```python
from build123d import *

# Parameters (mm, degrees)
ESTRUSIONE_ESTRUSIONE2_DEPTH = 1.6


with BuildPart() as part:
    # bordo2 → Estrusione-Estrusione2 (new body)
    with BuildSketch(Plane.XY):
        with BuildLine():
            Line((201, 97.893856635), (201, -7.091597346))
            ThreePointArc((201, -7.091597346), (198.656854249, -12.748451596), (193, -15.091597346))
            Line((193, -15.091597346), (117.750790543, -15.091597346))
            ThreePointArc((117.750790543, -15.091597346), (116.336576981, -14.505810909), (115.750790543, -13.091597346))
            Line((115.750790543, -13.091597346), (115.750790543, -12.967534141))
            ThreePointArc((115.750790543, -12.967534141), (115.127499694, -11.516785399), (113.64611863, -10.970275071))
            Line((113.64611863, -10.970275071), (0.928841556, -16.877537249))
            ThreePointArc((0.928841556, -16.877537249), (-0.145141858, -16.910699844), (-1.219558299, -16.897682863))
            Line((-1.219558299, -16.897682863), (-151.023233988, -11.861429997))
            ThreePointArc((-151.023233988, -11.861429997), (-156.505538032, -9.426954116), (-158.754433684, -3.865947122))
            Line((-158.754433684, -3.865947122), (-158.754433684, 95.67986032))
            Line((-158.754433684, 95.67986032), (-158.754433684, 110.187089821))
            ThreePointArc((-158.754433684, 110.187089821), (-154.068142183, 121.50079832), (-142.754433684, 126.187089821))
            Line((-142.754433684, 126.187089821), (-39, 126.187089821))
            ThreePointArc((-39, 126.187089821), (-33.343145751, 123.843944071), (-31, 118.187089821))
            Line((-31, 118.187089821), (-31, 105.006491693))
            ThreePointArc((-31, 105.006491693), (-28.802994968, 99.499655087), (-23.41868765, 97.017455415))
            Line((-23.41868765, 97.017455415), (-2.104671912, 95.900435182))
            ThreePointArc((-2.104671912, 95.900435182), (-0.623290849, 96.44694551), (0, 97.897694252))
            Line((0, 97.897694252), (0, 100.897694252))
            ThreePointArc((0, 100.897694252), (0.549251258, 102.274403403), (1.895328088, 102.894953321))
            Line((1.895328088, 102.894953321), (97.91868765, 107.927324355))
            ThreePointArc((97.91868765, 107.927324355), (103.302994968, 110.409524028), (105.5, 115.916360633))
            Line((105.5, 115.916360633), (105.5, 126))
            ThreePointArc((105.5, 126), (107.843145751, 131.656854249), (113.5, 134))
            Line((113.5, 134), (169.851790543, 134))
            ThreePointArc((169.851790543, 134), (172.680217668, 132.828427125), (173.851790543, 130))
            Line((173.851790543, 130), (173.851790543, 130.276535982))
            ThreePointArc((173.851790543, 130.276535982), (175.023363418, 127.448108857), (177.851790543, 126.276535982))
            Line((177.851790543, 126.276535982), (185, 126.276535982))
            ThreePointArc((185, 126.276535982), (196.313708499, 121.590244481), (201, 110.276535982))
            Line((201, 110.276535982), (201, 97.893856635))
        make_face()
    extrude(amount=ESTRUSIONE_ESTRUSIONE2_DEPTH)


solid = part.part
```
The listing builds one solid part. Answer for the finished solid, in the listing's coordinates (mm). A direction names the side the tool comes from. Round coordinates to 2 decimals unless told otherwise and drop trailing zeros. Loops run counter-clockwise (first coordinate to the right, second up) from the corner with the lowest first, then second, coordinate; pieces in that order, holes last.
Q1. Which of the six approach directions +Z, -Z, +X, -X, +Y, -Y give full straight-line access (tool end or side, diameter ignored) to faces 1 (the face through (103.244, 110.348, 0.789)), 2 (the face through (58.077, -13.883, 0.789)), 3 (the face through (-156.445, -9.489, 0.789))?
Q2. Find the intervals of material crossed by line 1 (X direction, y = 110, z = 1.55); line 2 (Y direction, x = 168, z = 0.5); line 3 (Y direction, x = -55.5, z = 0.5), in increasing order.
Q3. Section B-B, the plane x = 68.5 is taken. Determine the outline of the cut face in (y, z), then the cut area to 3 significant figures.
Q4. For a pull along X with two mould halves and no side action, classify faces 4 (the face through (24, 43, 0)), 5 (the face through (196.19, 121.71, 0.79)), 6 (the face through (-154.19, 121.38, 0.79)), 7 (the face through (-28.86, 99.56, 0.79)) as released by +X, released by -X, zero draft, split by the parting line, or undercut.
Q5. Given pin 1 Ø0.8 at (x, z) = (154.5, 1) entering from -Y; pin 2 Ø0.5 at (x, z) = (-116, 1) entering from +Y; pin 3 Ø0.8 at (x, z) = (180, 0.5) entering from +Y, each flat-ended and moving along its own axis, determine where each tip first touches the part or whether it passes through.
Q6. Section C-C, the plane x = -70 is taken. Determine the outline of the cut face in (y, z), then the cut area to 3 significant figures.
Completed:
1. face 1: +Z, -Z, +Y
1. face 2: +Z, -Z, -Y
1. face 3: +Z, -Z, -X, -Y
2. line 1: x = -158.75 to -31, 102.88 to 201
2. line 2: y = -15.09 to 134
2. line 3: y = -15.07 to 126.19
3. outline: (-13.34, 0) - (106.39, 0) - (106.39, 1.6) - (-13.34, 1.6) - close
3. area: 192 mm2
4. face 4: zero draft
4. face 5: released by +X
4. face 6: released by -X
4. face 7: undercut
5. pin 1: stops at y = -15.09
5. pin 2: stops at y = 126.19
5. pin 3: stops at y = 126.28
6. outline: (-14.59, 0) - (126.19, 0) - (126.19, 1.6) - (-14.59, 1.6) - close
6. area: 225 mm2
